Check sheet for the modelled part. Datum: model origin and axes. Units: mm. Face numbers are marked on the shaded views. Coordinates: 2 decimals unless noted, no trailing zeros. Loops run counter-clockwise (first coordinate to the right, second up) from the corner with the lowest first, then second, coordinate; pieces in that order, holes last. Notation, with made-up numbers: (38.5, -12) - (52.5, -12) arc R24 cw to (52.5, 23) - close; hole circle Ø3 at (48, 89.25). An arc over 180 degrees is marked (long way). Use a Markdown table: item, result. Add a question column.
1) Sectioned sample at B-B, the plane z = 6. Enter the section's corners in (x, y).
2) Sectioned sample at C-C, the plane x = 0. Enter the section's corners in (y, z), then the cut area to 3 significant figures.
3) Go/stop test with flat-tipped pins: P1, Ø5, axis at y = 47.5, z = 12, coming from the -X side; P2, Ø4, axis at y = 48, z = 4.5, coming from the +X side; P3, Ø12, axis at x = -48.5, z = 9.5, coming from the -Y side. Record where each tip stops, or that it passes through.
4) Sectioned sample at A-A, the plane y = 47. Enter the section's corners in (x, z), then the cut area to 3 significant figures.
5) Draft check along Y on the marked faces 1, 2 and 3. Enter one of: pulls with the +Y half, pulls with the -Y half, needs draft (parallel to the pull), parting line crosses it, or undercut.
6) Sectioned sample at D-D, the plane y = 112.5. Enter the section's corners in (x, z), then the cut area to 3 significant figures.
7) Thickness scan on line 1 (X direction, y = 7, z = 1.75); line 2 (X direction, y = 12.5, z = 11.5); line 3 (X direction, y = 46.5, z = 11.75). Record the ranges inside material, lowest first.
from build123d import *

# Parameters (mm, degrees)
F1_DEPTH = 20
F2_R     = 3


# Not quite as in the source:
# - a feature names something its author has since deleted; it is built from what else it names


with BuildPart() as f1:
    # F0 (on Top) → F1 (new body)
    with BuildSketch(Plane.XY):
        with BuildLine():
            Line((-153.2121218782, 14.4520842503), (-160.3632725747, 14.4520842503))
            ThreePointArc((-160.3632725747, 14.4520842503), (-127.3979918157, -21.6045066339), (-88.538816916, 8.0054918097))
            ThreePointArc((-88.538816916, 8.0054918097), (7.672936475, 88.5682564232), (88.5964468438, -7.3402729282))
            ThreePointArc((88.5964468438, -7.3402729282), (87.9631543537, -12.872197798), (86.984793992, -18.3536267309))
            ThreePointArc((86.984793992, -18.3536267309), (86.0838715562, -22.1985823397), (85.013080464, -25.9997336529))
            ThreePointArc((85.013080464, -25.9997336529), (84.2979595084, -36.2275225271), (87.887852798, -45.8312577069))
            ThreePointArc((87.887852798, -45.8312577069), (96.3394016955, -54.8865279313), (106.4780767567, -62.0022756507))
            ThreePointArc((106.4780767567, -62.0022756507), (116.2685705091, -67.06105094), (127.0920702884, -69.1339300658))
            ThreePointArc((127.0920702884, -69.1339300658), (157.854119606, -37.8760326334), (124.6599386157, -9.2141035549))
            ThreePointArc((124.6599386157, -9.2141035549), (124.7149682754, -8.4366277665), (124.7651490421, -7.6588239637))
            ThreePointArc((124.7651490421, -7.6588239637), (12.9161691706, 124.330899514), (-123.675215649, 18.1505105758))
            ThreePointArc((-123.675215649, 18.1505105758), (-136.3484686697, -0.431692042), (-153.2121218782, 14.4520842503))
        make_face()
        with BuildLine():
            ThreePointArc((127.83052, -30.8446834837), (133.6641509448, -33.2610525389), (136.08052, -39.0946834837))
            ThreePointArc((136.08052, -39.0946834837), (133.6641509448, -44.9283144285), (127.83052, -47.3446834837))
            ThreePointArc((127.83052, -47.3446834837), (121.9968890552, -44.9283144285), (119.58052, -39.0946834837))
            ThreePointArc((119.58052, -39.0946834837), (121.9968890552, -33.2610525389), (127.83052, -30.8446834837))
        make_face(mode=Mode.SUBTRACT)
    extrude(amount=F1_DEPTH)

    # F2
    f2_edges = [f1.edges().sort_by_distance(p)[0] for p in [
        (-160.363273, 14.452084, 10),
        (-153.212122, 14.452084, 10),
    ]]
    fillet(f2_edges, radius=F2_R)


solid = f1.part
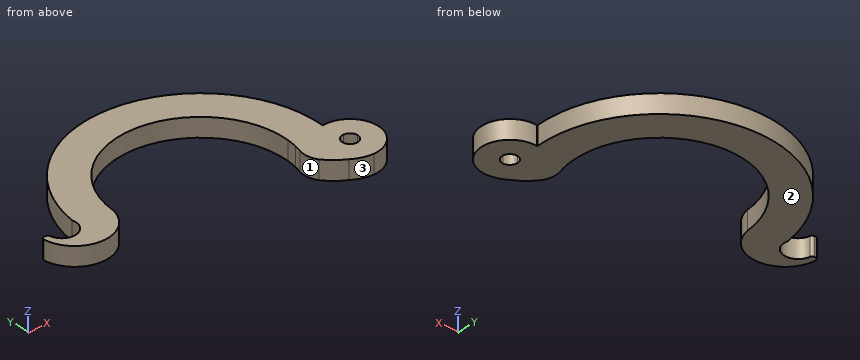
Solved:
| question | item | result |
|---|---|---|
| 1 | outline | (-160.22, 11.18) arc R36.2 ccw to (-88.54, 8.01) arc R88.9 cw (long way) to (85.01, -26) arc R24.17 ccw to (87.89, -45.83) arc R59.68 ccw to (106.48, -62) arc R38.44 ccw to (127.09, -69.13) arc R30.05 ccw (long way) to (124.66, -9.21) arc R125 ccw to (124.77, -7.66) arc R125 ccw to (-123.68, 18.15) arc R15 cw (long way) to (-153, 11.95) arc R3 ccw to (-155.96, 14.45) - (-157.23, 14.45) arc R3 ccw to start; hole circle Ø16.5 at (127.83, -39.09) |
| 2 | outline | (88.9, 0) - (125, 0) - (125, 20) - (88.9, 20) - close |
| 2 | area | 722 mm2 |
| 3 | P1 | stops at x = -116.62 |
| 3 | P2 | stops at x = 116.23 |
| 3 | P3 | stops at y = 70.24 |
| 4 | outline | (-115.83, 0) - (-75.46, 0) - (-75.46, 20) - (-115.83, 20) - close; (75.46, 0) - (115.83, 0) - (115.83, 20) - (75.46, 20) - close |
| 4 | area | 1,610 mm2 |
| 5 | face 1 | undercut |
| 5 | face 2 | needs draft |
| 5 | face 3 | pulls with the -Y half |
| 6 | outline | (-54.49, 0) - (54.49, 0) - (54.49, 20) - (-54.49, 20) - close |
| 6 | area | 2,180 mm2 |
| 7 | line 1 | x = -159.59 to -151.23, -125.19 to -88.74, 88.62 to 124.8 |
| 7 | line 2 | x = -160.04 to -153.15, -123.34 to -88.02, 88.02 to 124.37 |
| 7 | line 3 | x = -116.03 to -75.77, 75.77 to 116.03 |
